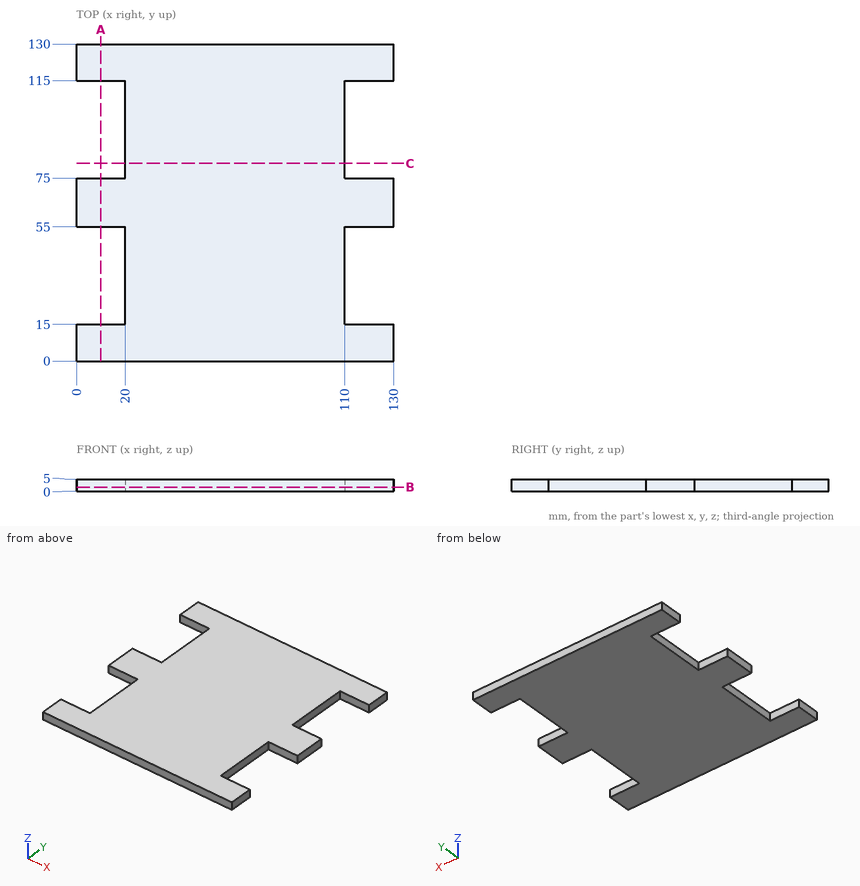
Answer from the drawing. Dimensions are ordinates in mm from the lowest x, y and z of the part. Give positions to 0.01 mm unless a question says otherwise; leave off trailing zeros. Order: outer loops, then holes, each group sorted by start corner. A loop starts at its lowest first (then second) coordinate and runs counter-clockwise, first axis right, second up.
(1) Find section C-C (y = 81). Give the vertices of the cut face in (x, z), plus the area to 3 significant figures.
(2) Find section A-A (x = 10). Give the vertices of the cut face in (y, z), plus the area to 3 significant figures.
(3) Straight lines are drawn through the part: L1, parallel to Y at x = 10, z = 0.9; L2, parallel to X at y = 105, z = 2.8. For each, find the intervals that lie inside material, in ascending order.
(4) Given pin 1 (2.5 mm diameter, centred on y = 99, z = 2, fed in from +X); pin 2 (2.5 mm diameter, centred on y = 29, z = 2, fed in from -X), each flat-ended and moving along its own axis, determine where each tip first touches the part or whether it passes through.
(5) Find section B-B (z = 1.7). Give the vertices of the cut face in (x, y).
Result sheet:
1. outline: (20, 0) - (110, 0) - (110, 5) - (20, 5) - close
1. area: 450 mm2
2. outline: (0, 0) - (15, 0) - (15, 5) - (0, 5) - close; (55, 0) - (75, 0) - (75, 5) - (55, 5) - close; (115, 0) - (130, 0) - (130, 5) - (115, 5) - close
2. area: 250 mm2
3. L1: y = 0 to 15, 55 to 75, 115 to 130
3. L2: x = 20 to 110
4. pin 1: stops at x = 110
4. pin 2: stops at x = 20
5. outline: (0, 0) - (130, 0) - (130, 15) - (110, 15) - (110, 55) - (130, 55) - (130, 75) - (110, 75) - (110, 115) - (130, 115) - (130, 130) - (0, 130) - (0, 115) - (20, 115) - (20, 75) - (0, 75) - (0, 55) - (20, 55) - (20, 15) - (0, 15) - close
